```python
from build123d import *

# Parameters (mm, degrees)
F0_W     = 330
F0_H     = 20
F0_R     = 4
F1_DEPTH = 3
F2_DEPTH = 5
F4_R     = 10
F5_DEPTH = 3


with BuildPart() as f1:
    # F0 (on Right) → F1 (new body)
    with BuildSketch(Plane.YZ):
        with Locations((165, 10)):
            Rectangle(F0_W, F0_H)
        with Locations((30, 10)):
            Circle(F0_R, mode=Mode.SUBTRACT)
        with Locations((320, 10)):
            Circle(F0_R, mode=Mode.SUBTRACT)
        with Locations((320, 10)):
            Circle(F0_R)
    extrude(amount=F1_DEPTH)

    # F0 (on Right) → F2 (join)
    with BuildSketch(Plane.YZ):
        with Locations((320, 10)):
            Circle(F0_R)
    extrude(amount=-F2_DEPTH)

    # F4 (on offset) → F5 (join)
    with BuildSketch(Plane.YZ.offset(-5)):
        with Locations((320, 10)):
            Circle(F4_R)
    extrude(amount=-F5_DEPTH)


solid = f1.part
```
Input: part model. Units: mm. Frame: model coordinates. A direction names the side the tool comes from. Give positions to 0.01 mm unless a question says otherwise; leave off trailing zeros. Order: outer loops, then holes, each group sorted by start corner. A loop starts at its lowest first (then second) coordinate and runs counter-clockwise, first axis right, second up. Notation, with made-up numbers: M -14.5,66 L 23.5,66 A13 cw 23.5,90 Z; hole C -27,66.25 d10. An arc over 180 degrees is marked long. Return JSON: item names as keys, results as strings.
1) Access query for faces 4 (the face through (-2, 316, 10)), 5 (the face through (1, 26, 10)). Directions: +Z, -Z, +X, -X, +Y, -Y. A direction counts if a zero-diameter tool reaches every point of the face in a straight line with its end or side. Return the directions, or none.
Taken from the geometry:
{"face 4": "none", "face 5": "+X, -X"}
2) Section query C-C on y = 320. Output: boundary loops of the cut face in (x, z), and give its area (3 significant figures).
Taken from the geometry:
{"outline": "M -8,0 L -5,0 L -5,6 L 0,6 L 0,0 L 3,0 L 3,20 L 0,20 L 0,14 L -5,14 L -5,20 L -8,20 Z", "area": "160 mm2"}
3) Mould query, pull axis X, two halves, no side actions, for faces 1 (the face through (-6, 312, 4)), 2 (the face through (-5, 319.9, 5.7)), 3 (the face through (3, 163, 10)). Classes: released by +X, released by -X, zero draft, split by the parting line, or undercut.
Taken from the geometry:
{"face 1": "zero draft", "face 2": "undercut", "face 3": "released by +X"}
4) Section query D-D on x = -3.25. Output: boundary loops of the cut face in (y, z).
Taken from the geometry:
{"outline": "C 320,10 d8"}
5) Section query A-A on y = 30. Output: boundary loops of the cut face in (x, z).
Taken from the geometry:
{"outline": "M 0,0 L 3,0 L 3,6 L 0,6 Z; M 0,14 L 3,14 L 3,20 L 0,20 Z"}
6) Contact query for flat-ended pins moving along their axis: pin 1 (4 mm diameter, centred on x = -6, z = 4, fed in from -Y); pin 2 (2 mm diameter, centred on y = 233.5, z = 5.5, fed in from -X). Output: stop coordinate, or through.
Taken from the geometry:
{"pin 1": "stops at y = 310.83", "pin 2": "stops at x = 0"}
7) Section query B-B on z = 10. Output: boundary loops of the cut face in (x, y).
Taken from the geometry:
{"outline": "M -8,310 L -5,310 L -5,316 L 0,316 L 0,34 L 3,34 L 3,330 L 0,330 L 0,324 L -5,324 L -5,330 L -8,330 Z; M 0,0 L 3,0 L 3,26 L 0,26 Z"}
8) Line query: L1, parallel to Z at x = 2.25, y = 30; L2, parallel to X at y = 244, z = 5.5; L3, parallel to Y at x = -6.5, z = 8.25. Output: solid intervals per line, ascending. Write a range as [from, to].
Taken from the geometry:
{"L1": "z = [0, 6], [14, 20]", "L2": "x = [0, 3]", "L3": "y = [310.15, 329.85]"}
